Read the model definition and answer for the solid it produces. Units are mm, in the model's axes. Face numbers are marked on the shaded views. Round coordinates to 2 decimals unless told otherwise and drop trailing zeros. Write each loop counter-clockwise with the first axis right and the second up, starting at its lowest first coordinate (ties: lowest second). Pieces come first, ordered by that corner, then holes.
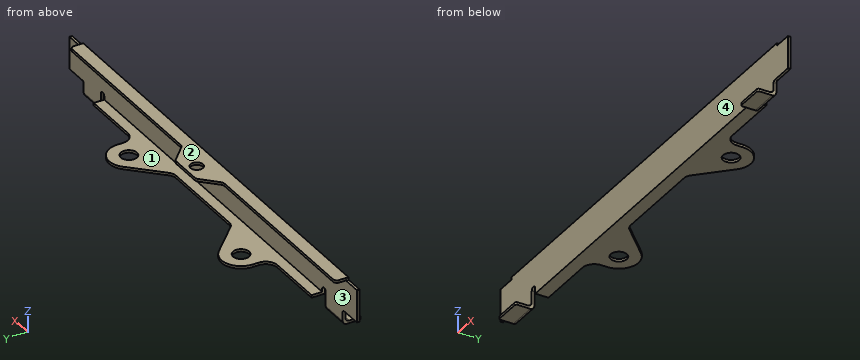
from build123d import *

# Parameters (mm, degrees)
BOSS_EXTRUDE1_DEPTH = 1.651
SKETCH2_W           = 18.415
SKETCH2_H           = 1.651
BOSS_EXTRUDE2_DEPTH = 10.287
FILLET1_R           = 2.54
FILLET3_R           = 1.27
SKETCH4_W           = 235.6739
SKETCH4_H           = 1.651
SKETCH4_W_2         = 286.8803
BOSS_EXTRUDE3_DEPTH = 30.861
SKETCH5_R           = 4.0005
CUT_EXTRUDE2_DEPTH  = 2.54
FILLET4_R           = 2.54
SKETCH11_R          = 5.207
CUT_EXTRUDE3_DEPTH  = 7.62


with BuildPart() as part:
    # Sketch1 → Boss-Extrude1 (new body)
    with BuildSketch(Plane(origin=(0, 0, 0), x_dir=(1, 0, 0), z_dir=(0, 1, 0))):
        with BuildLine():
            Line((117.83695, 8.5725), (117.83695, 12.1285))
            Line((117.83695, 12.1285), (117.186124302, 12.1285))
            Line((117.186124302, 12.1285), (-117.186124302, 12.1285))
            Line((-117.186124302, 12.1285), (-117.83695, 12.1285))
            Line((-117.83695, 12.1285), (-117.83695, 8.5725))
            ThreePointArc((-117.83695, 8.5725), (-119.74195, 6.6675), (-121.64695, 8.5725))
            Line((-121.64695, 8.5725), (-121.64695, 12.1285))
            Line((-121.64695, 12.1285), (-121.64695, 20.2565))
            Line((-121.64695, 20.2565), (-140.06195, 20.2565))
            Line((-140.06195, 20.2565), (-140.06195, 12.1285))
            Line((-140.06195, 12.1285), (-140.06195, 11.7475))
            ThreePointArc((-140.06195, 11.7475), (-140.433924388, 10.849474388), (-141.33195, 10.4775))
            Line((-141.33195, 10.4775), (-143.44015, 10.4775))
            Line((-143.44015, 10.4775), (-155.37815, 10.4775))
            Line((-155.37815, 10.4775), (-155.37815, -10.4775))
            Line((-155.37815, -10.4775), (-144.20215, -10.4775))
            ThreePointArc((-144.20215, -10.4775), (-143.663334633, -10.700684633), (-143.44015, -11.2395))
            Line((-143.44015, -11.2395), (-143.44015, -12.1285))
            Line((-143.44015, -12.1285), (143.44015, -12.1285))
            Line((143.44015, -12.1285), (143.44015, -11.2395))
            ThreePointArc((143.44015, -11.2395), (143.663334633, -10.700684633), (144.20215, -10.4775))
            Line((144.20215, -10.4775), (155.37815, -10.4775))
            Line((155.37815, -10.4775), (155.37815, 10.4775))
            Line((155.37815, 10.4775), (143.44015, 10.4775))
            Line((143.44015, 10.4775), (141.33195, 10.4775))
            ThreePointArc((141.33195, 10.4775), (140.433924388, 10.849474388), (140.06195, 11.7475))
            Line((140.06195, 11.7475), (140.06195, 12.1285))
            Line((140.06195, 12.1285), (140.06195, 20.2565))
            Line((140.06195, 20.2565), (121.64695, 20.2565))
            Line((121.64695, 20.2565), (121.64695, 12.1285))
            Line((121.64695, 12.1285), (121.64695, 8.5725))
            ThreePointArc((121.64695, 8.5725), (119.74195, 6.6675), (117.83695, 8.5725))
        make_face()
    extrude(amount=BOSS_EXTRUDE1_DEPTH)

    # Sketch2 → Boss-Extrude2 (add)
    with BuildSketch(Plane.XZ):
        with Locations((-130.85445, -19.431)):
            Rectangle(SKETCH2_W, SKETCH2_H)
        with Locations((130.85445, -19.431)):
            Rectangle(SKETCH2_W, SKETCH2_H)
    extrude(amount=BOSS_EXTRUDE2_DEPTH)

    # Fillet1
    fillet1_edges = [part.edges().sort_by_distance(p)[0] for p in [
        (130.85445, 1.651, -20.2565),
        (-130.85445, 1.651, -20.2565),
        (-130.85445, 0, -18.6055),
        (130.85445, 0, -18.6055),
    ]]
    fillet(fillet1_edges, radius=FILLET1_R)

    # Fillet3
    fillet3_edges = [part.edges().sort_by_distance(p)[0] for p in [
        (-140.06195, -10.287, -19.431),
        (-121.64695, -10.287, -19.431),
        (140.06195, -10.287, -19.431),
        (121.64695, -10.287, -19.431),
    ]]
    fillet(fillet3_edges, radius=FILLET3_R)

    # Sketch4 → Boss-Extrude3 (add)
    with BuildSketch(Plane(origin=(0, 1.651, 0), x_dir=(1, 0, 0), z_dir=(0, 1, 0))):
        with Locations((0, 11.303)):
            Rectangle(SKETCH4_W, SKETCH4_H)
        with Locations((0, -11.303)):
            Rectangle(SKETCH4_W_2, SKETCH4_H)
    extrude(amount=BOSS_EXTRUDE3_DEPTH)

    # Sketch5 → Cut-Extrude2 (cut)
    with BuildSketch(Plane.XY.offset(12.1285)):
        with Locations((0, 12.2555)):
            Circle(SKETCH5_R)
        Polygon((143.44015, 8.4582), (22.43455, 8.4582), (11.1125, 19.431), (-11.1125, 19.431), (-22.43455, 8.4582), (-143.44015, 8.4582), (-143.44015, 32.512), (143.44015, 32.512), align=None)
    extrude(amount=-CUT_EXTRUDE2_DEPTH, mode=Mode.SUBTRACT)

    # Fillet4
    fillet4_edges = [part.edges().sort_by_distance(p)[0] for p in [
        (143.44015, 8.4582, 11.303),
        (22.43455, 8.4582, 11.303),
        (11.1125, 19.431, 11.303),
        (-11.1125, 19.431, 11.303),
        (-22.43455, 8.4582, 11.303),
        (-143.44015, 8.4582, 11.303),
    ]]
    fillet(fillet4_edges, radius=FILLET4_R)

    # Sketch11 → Cut-Extrude3 (cut)
    with BuildSketch(Plane(origin=(0, 0, -12.1285), x_dir=(-1, 0, 0), z_dir=(0, 0, -1))):
        with Locations((60.68695, 19.812)):
            Circle(SKETCH11_R)
        with Locations((-60.68695, 19.812)):
            Circle(SKETCH11_R)
        with BuildLine():
            Line((81.00695, 8.4582), (117.83695, 8.4582))
            Line((117.83695, 8.4582), (117.83695, 32.512))
            Line((117.83695, 32.512), (60.68695, 32.512))
            ThreePointArc((60.68695, 32.512), (69.667206121, 28.792256121), (73.38695, 19.812))
            Line((73.38695, 19.812), (73.38695, 16.0782))
            ThreePointArc((73.38695, 16.0782), (75.618796327, 10.690046327), (81.00695, 8.4582))
        make_face()
        with BuildLine():
            Line((-28.742381637, 8.4582), (0, 8.4582))
            Line((0, 8.4582), (28.742381637, 8.4582))
            ThreePointArc((28.742381637, 8.4582), (31.172421432, 8.941564969), (33.232509697, 10.318071939))
            Line((33.232509697, 10.318071939), (51.706693879, 28.792256121))
            ThreePointArc((51.706693879, 28.792256121), (55.826870409, 31.545270063), (60.68695, 32.512))
            Line((60.68695, 32.512), (-60.68695, 32.512))
            ThreePointArc((-60.68695, 32.512), (-55.826870409, 31.545270063), (-51.706693879, 28.792256121))
            Line((-51.706693879, 28.792256121), (-33.232509697, 10.318071939))
            ThreePointArc((-33.232509697, 10.318071939), (-31.172421432, 8.941564969), (-28.742381637, 8.4582))
        make_face()
        with BuildLine():
            Line((-117.83695, 32.512), (-117.83695, 8.4582))
            Line((-117.83695, 8.4582), (-81.00695, 8.4582))
            ThreePointArc((-81.00695, 8.4582), (-75.618796327, 10.690046327), (-73.38695, 16.0782))
            Line((-73.38695, 16.0782), (-73.38695, 19.812))
            ThreePointArc((-73.38695, 19.812), (-69.667206121, 28.792256121), (-60.68695, 32.512))
            Line((-60.68695, 32.512), (-117.83695, 32.512))
        make_face()
    extrude(amount=-CUT_EXTRUDE3_DEPTH, mode=Mode.SUBTRACT)


solid = part.part
Q1. Flat-ended cylindrical pins translate along their axes: pin 1 Ø0.8 at (x, z) = (104.5, 11.5) entering from +Y; pin 2 Ø3 at (y, z) = (-2, -17) entering from -X; pin 3 Ø8.5 at (x, z) = (74, 3) entering from -Y; pin 4 Ø10 at (y, z) = (1.5, -13) entering from -X. Find the tip coordinate at first contact, or state that the pin passes through.
Verdict:
pin 1: stops at y = 8.46
pin 2: stops at x = -140.06
pin 3: stops at y = 0
pin 4: stops at x = -155.38
Q2. Section A-A (x = 0) is taken. Determine the outline of the cut face in (y, z) (1 decimal), then the cut area to 3 significant figures.
Verdict:
outline: (0, -12.1) - (8.5, -12.1) - (8.5, -10.5) - (1.7, -10.5) - (1.7, 10.5) - (8.3, 10.5) - (8.3, 12.1) - (0, 12.1) - close; (16.3, 10.5) - (19.4, 10.5) - (19.4, 12.1) - (16.3, 12.1) - close
area: 67.4 mm2
Q3. Determine the mould class of the marked faces 1, 2, 3 and 4 for opening direction Z: pulls with the +Z half, pulls with the -Z half, needs draft (parallel to the pull), parting line crosses it, or undercut.
Verdict:
face 1: undercut
face 2: pulls with the +Z half
face 3: undercut
face 4: needs draft
Q4. Section C-C (x = -37) is taken. Determine the outline of the cut face in (y, z).
Verdict:
outline: (0, -12.13) - (14.09, -12.13) - (14.09, -10.48) - (1.65, -10.48) - (1.65, 10.48) - (8.46, 10.48) - (8.46, 12.13) - (0, 12.13) - close
Q5. Straight lines are drawn through the part: probe 1 along Y at (x, z) = (0, 11.55) (3 decimals); probe 2 along Z at (x, y) = (-14.5, 1); probe 3 along Z at (x, y) = (7, 12). For each, find the intervals that lie inside material, in ascending order.
Verdict:
probe 1: y = 0 to 8.255, 16.256 to 19.431
probe 2: z = -12.13 to 12.13
probe 3: z = 10.48 to 12.13
Q6. Section B-B (z = -1) is taken. Determine the outline of the cut face in (x, y), then the cut area to 3 significant figures.
Verdict:
outline: (-155.38, 0) - (155.38, 0) - (155.38, 1.65) - (-155.38, 1.65) - close
area: 513 mm2
